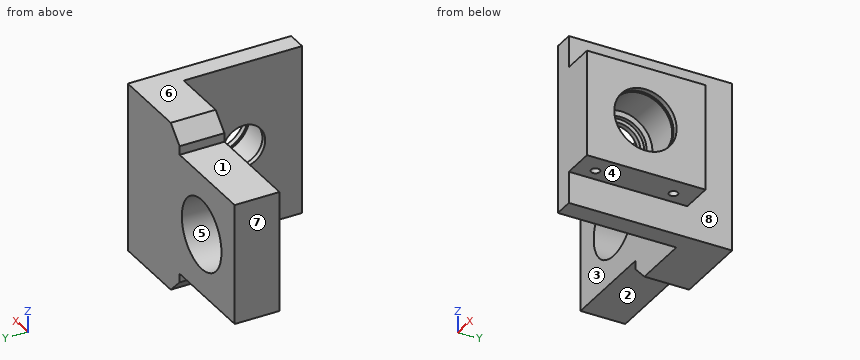
from build123d import *

# Parameters (mm, degrees)
F0_R     = 18
F1_DEPTH = 23
F2_DEPTH = 83.8
F3_START = 23
F0_W     = 16.5
F0_H     = 54.5
F3_DEPTH = 60.8
F6_SIZE2 = 8
F6_SIZE  = 8
F8_D     = 4.4
F8_DEPTH = 8
F8_TIP   = 1.3218933619


with BuildPart() as f1:
    # F0 (on Front) → F1 (new body)
    with BuildSketch(Plane.XZ):
        Polygon((-30, 31), (-30, -31), (20, -31), (20, -43.5), (57, -43.5), (57, 43.5), (20, 43.5), (20, 31), align=None)
        Circle(F0_R, mode=Mode.SUBTRACT)
    extrude(amount=F1_DEPTH)

    # F0 (on Front) → F2 (join)
    with BuildSketch(Plane.XZ):
        Polygon((57, 43.5), (57, -43.5), (67, -43.5), (67, -27.25), (67, 27.25), (67, 43.5), align=None)
    extrude(amount=F2_DEPTH)

    # F0 (on Front) → F3 (join)
    with BuildSketch(Plane.XZ.offset(F3_START)):
        with Locations((75.25, 0)):
            Rectangle(F0_W, F0_H)
    extrude(amount=F3_DEPTH)

    # F4 (on Top) → F5 (revolve, cut)
    with BuildSketch(Plane.XY):
        Polygon((57, -53.82), (57, -64.82), (59.5, -64.82), (59.5, -66.82), (61.5, -66.82), (61.5, -69.82), (79.5, -69.82), (79.5, -70.67), (80.8, -70.67), (80.8, -69.82), (83.5, -69.82), (83.5, -53.82), align=None)
    revolve(axis=Axis((70.25, -53.82, 0), (-1, 0, 0)), mode=Mode.SUBTRACT)

    # F6
    f6_edges = [f1.edges().sort_by_distance(p)[0] for p in [
        (20, -11.5, 43.5),
        (20, -11.5, -43.5),
    ]]
    chamfer(f6_edges, length=F6_SIZE, length2=F6_SIZE2)

    # F8
    with Locations(Plane(origin=(0, 0, -27.25), x_dir=(1, 0, 0), z_dir=(0, 0, -1))):
        with Locations((73.5, 73.82), (73.5, 33.82)):
            Hole(F8_D / 2, depth=F8_DEPTH)
            with Locations((0, 0, -(F8_DEPTH + F8_TIP / 2))):  # 118° drill point
                Cone(0, F8_D / 2, F8_TIP, mode=Mode.SUBTRACT)


solid = f1.part
Work out the finished part from the listing and answer in its coordinate system (mm). Face numbers are marked on the shaded views. A direction names the side the tool comes from. Give positions to 0.01 mm unless a question says otherwise; leave off trailing zeros. Loops run counter-clockwise (first coordinate to the right, second up) from the corner with the lowest first, then second, coordinate; pieces in that order, holes last. Notation, with made-up numbers: (-33, -12.5) -> (13, -12.5) arc R12 ccw to (13, 8.5) -> close; hole circle Ø4 at (-16.5, 50). An arc over 180 degrees is marked (long way). Use a Markdown table: item, result. Add a question column.
1. For the marked faces 1, 2, 3 and 4, determine the directions among +Z, -Z, +X, -X, +Y, -Y from which every point of the face is accessible in a straight line to the end or side of a thin tool.
2. Find the intervals of material crossed by probe 1 along Z at (x, y) = (0, -14); probe 2 along Y at (x, z) = (73, -24); probe 3 along Z at (x, y) = (72, -54), in increasing order.
3. Section B-B on z = 0 is taken. State how many separate pieces and enclosed holes the cut face has, and give its area (3 significant figures).
4. Section A-A on x = 0 is taken. Determine the outline of the cut face in (y, z).
5. Flat-ended cylindrical pins translate along their axes: pin 1 Ø2 at (y, z) = (-15.5, -34) entering from -X; pin 2 Ø17 at (y, z) = (-48, 2.5) entering from +X; pin 3 Ø2.5 at (x, y) = (73.5, -33.82) entering from +Z. Find the tip coordinate at first contact, or state that the pin passes through.
6. Section C-C on y = -53.82 is taken. Determine the outline of the cut face in (x, z), and give its area (3 significant figures).
7. Determine the mould class of the marked faces 5, 6, 7 and 8 for opening direction X: released by +X, released by -X, zero draft, split by the parting line, or undercut.
8. Section D-D on z = 21.5 is taken. Determine the outline of the cut face in (x, y).
Results below:
| question | item | result |
|---|---|---|
| 1 | face 1 | +Z, -X, +Y, -Y |
| 1 | face 2 | -Z, -X, +Y, -Y |
| 1 | face 3 | +Z, -Z, -X, -Y |
| 1 | face 4 | -Z, +X, +Y, -Y |
| 2 | probe 1 | z = -31 to -18, 18 to 31 |
| 2 | probe 2 | y = -83.8 to -75.96, -71.68 to -35.96, -31.68 to -23 |
| 2 | probe 3 | z = -27.25 to -16, 16 to 27.25 |
| 3 | separate pieces | 3 |
| 3 | enclosed holes | 0 |
| 3 | area | 2,200 mm^2 |
| 4 | outline | (-23, -31) -> (0, -31) -> (0, -18) -> (-23, -18) -> close; (-23, 18) -> (0, 18) -> (0, 31) -> (-23, 31) -> close |
| 5 | pin 1 | stops at x = 20 |
| 5 | pin 2 | stops at x = 61.5 |
| 5 | pin 3 | stops at z = 27.25 |
| 6 | outline | (57, -43.5) -> (67, -43.5) -> (67, -27.25) -> (83.5, -27.25) -> (83.5, -16) -> (80.8, -16) -> (80.8, -16.85) -> (79.5, -16.85) -> (79.5, -16) -> (61.5, -16) -> (61.5, -13) -> (59.5, -13) -> (59.5, -11) -> (57, -11) -> close; (57, 11) -> (59.5, 11) -> (59.5, 13) -> (61.5, 13) -> (61.5, 16) -> (79.5, 16) -> (79.5, 16.85) -> (80.8, 16.85) -> (80.8, 16) -> (83.5, 16) -> (83.5, 27.25) -> (67, 27.25) -> (67, 43.5) -> (57, 43.5) -> close |
| 6 | area | 956 mm^2 |
| 7 | face 5 | undercut |
| 7 | face 6 | zero draft |
| 7 | face 7 | released by -X |
| 7 | face 8 | released by +X |
| 8 | outline | (-30, -23) -> (57, -23) -> (57, -83.8) -> (83.5, -83.8) -> (83.5, -23) -> (67, -23) -> (67, 0) -> (-30, 0) -> close |
